Input: part model. Units: mm. Frame: model coordinates. A direction names the side the tool comes from. Coordinates: 2 decimals unless noted, no trailing zeros. Loops run counter-clockwise (first coordinate to the right, second up) from the corner with the lowest first, then second, coordinate; pieces in that order, holes last. Notation, with made-up numbers: (2, 78.5) -> (11, 78.5) arc R15 ccw to (11, 96.5) -> close; hole circle Ø1 at (18.25, 22.25). An arc over 180 degrees is marked (long way). Answer as a JSON object with one key per item and string values.
from build123d import *

# Parameters (mm, degrees)
ESQUISSE1_W                  = 41
ESQUISSE1_H                  = 46
ESQUISSE1_R                  = 2.25
ESQUISSE1_R_2                = 1
BOSS_EXTRU_1_DEPTH           = 30
ENL_V_START                  = 30
ESQUISSE2_W                  = 7
ESQUISSE2_H                  = 46
ENL_V_MAT_EXTRU_1_DEPTH      = 14
ENL_V_MAT_EXTRU_3_DEPTH      = 28.002906878
ENL_V_MAT_EXTRU_3_DEPTH_BACK = 44.002906878
ENL_V_MAT_EXTRU_3_START      = 16
ESQUISSE2_3_R                = 3
ESQUISSE3_W                  = 33.5
ESQUISSE3_H                  = 38
ENL_V_MAT_EXTRU_4_DEPTH      = 28
ESQUISSE4_W                  = 30
ESQUISSE4_H                  = 0.997507574
BOSS_EXTRU_2_DEPTH           = 1
CONG_1_R                     = 2
CONG_2_R                     = 2


# Some blends are built 0.0001 mm under size
with BuildPart() as part:
    # Esquisse1 → Boss.-Extru.1 (new body)
    with BuildSketch(Plane(origin=(0, 0, 0), x_dir=(1, 0, 0), z_dir=(0, 1, 0))):
        Rectangle(ESQUISSE1_W, ESQUISSE1_H)
        with Locations(Location((5.4, 0, 0), (0, 0, 270))):
            Circle(ESQUISSE1_R, mode=Mode.SUBTRACT)
        with Locations(Location((-1.85, 0, 0), (0, 0, 270))):
            Circle(ESQUISSE1_R_2, mode=Mode.SUBTRACT)
        with Locations(Location((12.65, 0, 0), (0, 0, 270))):
            Circle(ESQUISSE1_R_2, mode=Mode.SUBTRACT)
    extrude(amount=BOSS_EXTRU_1_DEPTH)

    # Esquisse2 → Enlèv. mat.-Extru.1 (cut)
    with BuildSketch(Plane(origin=(0, 0, 0), x_dir=(1, 0, 0), z_dir=(0, 1, 0)).offset(ENL_V_START)):
        with Locations((-17, 0)):
            Rectangle(ESQUISSE2_W, ESQUISSE2_H)
    extrude(amount=-ENL_V_MAT_EXTRU_1_DEPTH, mode=Mode.SUBTRACT)

    # Esquisse2<3> → Enlèv. mat.-Extru.3 (cut, two sides: drawn at the far end of the back side and taken through both)
    with BuildSketch(Plane(origin=(0, 0, 0), x_dir=(1, 0, 0), z_dir=(0, 1, 0)).offset(ENL_V_MAT_EXTRU_3_START - ENL_V_MAT_EXTRU_3_DEPTH_BACK)):
        with Locations(Location((-17, -8.75, 0), (0, 0, 90))):
            Circle(ESQUISSE2_3_R)
        with Locations(Location((-17, 8.75, 0), (0, 0, 90))):
            Circle(ESQUISSE2_3_R)
    extrude(amount=ENL_V_MAT_EXTRU_3_DEPTH + ENL_V_MAT_EXTRU_3_DEPTH_BACK, mode=Mode.SUBTRACT)

    # Esquisse3 → Enlèv. mat.-Extru.4 (cut)
    with BuildSketch(Plane(origin=(0, 0, 0), x_dir=(1, 0, 0), z_dir=(0, 1, 0))):
        with Locations((3.75, 0)):
            Rectangle(ESQUISSE3_W, ESQUISSE3_H)
    extrude(amount=ENL_V_MAT_EXTRU_4_DEPTH, mode=Mode.SUBTRACT)

    # Esquisse4 → Boss.-Extru.2 (add)
    with BuildSketch(Plane(origin=(0, 0, 0), x_dir=(1, 0, 0), z_dir=(0, 1, 0))):
        with Locations((5.5, -21)):
            Rectangle(ESQUISSE4_W, ESQUISSE4_H)
        with Locations((5.5, 21)):
            Rectangle(ESQUISSE4_W, ESQUISSE4_H)
    extrude(amount=-BOSS_EXTRU_2_DEPTH)

    # Congé1
    # the kernel refuses this fillet: 2 mm, written as the material it takes off along each edge
    with BuildSketch(Plane(origin=(-11.5, 28, -21), x_dir=(-1, 0, 0), z_dir=(0, 0, -1))) as cong_1_piece_1_section:
        Polygon((0, 0), (CONG_1_R, 0), (CONG_1_R, CONG_1_R), (0, CONG_1_R), align=None)
    cong_1_piece_1 = extrude(amount=CONG_1_R, mode=Mode.PRIVATE)
    cong_1_piece_1 = cong_1_piece_1 - Plane(origin=(-11.5, 28, -21), x_dir=(0.7071067811865475, -0.7071067811865475, 0), z_dir=(0, 0, -1)) * Sphere(CONG_1_R, mode=Mode.PRIVATE)
    add(cong_1_piece_1, mode=Mode.SUBTRACT)
    with BuildSketch(Plane(origin=(-18.5, 14, -21), x_dir=(0, 1, 0), z_dir=(-1, 0, 0))) as cong_1_piece_2_section:
        Polygon((0, 0), (CONG_1_R, 0), (CONG_1_R, CONG_1_R), (0, CONG_1_R), align=None)
    cong_1_piece_2 = extrude(amount=CONG_1_R, mode=Mode.PRIVATE)
    cong_1_piece_2 = cong_1_piece_2 - Plane(origin=(-18.5, 14, -21), x_dir=(0, -0.7071067811865475, 0.7071067811865475), z_dir=(-1, 0, 0)) * Sphere(CONG_1_R, mode=Mode.PRIVATE)
    add(cong_1_piece_2, mode=Mode.SUBTRACT)
    with BuildSketch(Plane(origin=(-11.5, 28, 21), x_dir=(-1, 0, 0), z_dir=(0, 0, 1))) as cong_1_piece_3_section:
        Polygon((0, 0), (CONG_1_R, 0), (CONG_1_R, -CONG_1_R), (0, -CONG_1_R), align=None)
    cong_1_piece_3 = extrude(amount=CONG_1_R, mode=Mode.PRIVATE)
    cong_1_piece_3 = cong_1_piece_3 - Plane(origin=(-11.5, 28, 21), x_dir=(0.7071067811865475, -0.7071067811865475, 0), z_dir=(0, 0, 1)) * Sphere(CONG_1_R, mode=Mode.PRIVATE)
    add(cong_1_piece_3, mode=Mode.SUBTRACT)
    with BuildSketch(Plane(origin=(-18.5, 14, 21), x_dir=(-1, 0, 0), z_dir=(0, 0, 1))) as cong_1_piece_4_section:
        Polygon((0, 0), (CONG_1_R, 0), (CONG_1_R, -CONG_1_R), (0, -CONG_1_R), align=None)
    cong_1_piece_4 = extrude(amount=CONG_1_R, mode=Mode.PRIVATE)
    cong_1_piece_4 = cong_1_piece_4 - Plane(origin=(-18.5, 14, 21), x_dir=(0.7071067811865475, -0.7071067811865475, 0), z_dir=(0, 0, 1)) * Sphere(CONG_1_R, mode=Mode.PRIVATE)
    add(cong_1_piece_4, mode=Mode.SUBTRACT)
    with BuildSketch(Plane(origin=(-11.5, 30, -23), x_dir=(0, 0, 1), z_dir=(1, 0, 0))) as cong_1_piece_5:
        with BuildLine():
            CenterArc((CONG_1_R, CONG_1_R), CONG_1_R, 180, 90)
            Line((0, CONG_1_R), (0, 0))
            Line((0, 0), (CONG_1_R, 0))
        make_face()
    extrude(amount=37, mode=Mode.SUBTRACT)
    with BuildSketch(Plane(origin=(-20.5, -5, -23), x_dir=(0, 0, 1), z_dir=(0, 1, 0)), Plane(origin=(-20.5, -5, 23), x_dir=(1, 0, 0), z_dir=(0, 1, 0))) as cong_1_piece_6:
        with BuildLine():
            CenterArc((CONG_1_R, CONG_1_R), CONG_1_R, 180, 90)
            Line((0, CONG_1_R), (0, 0))
            Line((0, 0), (CONG_1_R, 0))
        make_face()
    extrude(amount=19, mode=Mode.SUBTRACT)
    with BuildSketch(Plane(origin=(25.5, 30, 23), x_dir=(0, -1, 0), z_dir=(-1, 0, 0))) as cong_1_piece_7:
        with BuildLine():
            CenterArc((CONG_1_R, -CONG_1_R), CONG_1_R, 90, 90)
            Line((0, -CONG_1_R), (0, 0))
            Line((0, 0), (CONG_1_R, 0))
        make_face()
    extrude(amount=37, mode=Mode.SUBTRACT)
    with BuildSketch(Plane(origin=(-13.5, 16, 23), x_dir=(0, -1, 0), z_dir=(-1, 0, 0))) as cong_1_piece_8:
        with BuildLine():
            CenterArc((CONG_1_R, -CONG_1_R), CONG_1_R, 90, 90)
            Line((0, -CONG_1_R), (0, 0))
            Line((0, 0), (CONG_1_R, 0))
        make_face()
    extrude(amount=5, mode=Mode.SUBTRACT)
    with BuildSketch(Plane(origin=(-13.5, 28, 23), x_dir=(1, 0, 0), z_dir=(0, -1, 0)), Plane(origin=(-13.5, 28, -23), x_dir=(0, 0, 1), z_dir=(0, -1, 0))) as cong_1_piece_9:
        with BuildLine():
            CenterArc((CONG_1_R, -CONG_1_R), CONG_1_R, 90, 90)
            Line((0, -CONG_1_R), (0, 0))
            Line((0, 0), (CONG_1_R, 0))
        make_face()
    extrude(amount=12, mode=Mode.SUBTRACT)
    with BuildSketch(Plane(origin=(-20.5, 16, 21), x_dir=(0, -1, 0), z_dir=(0, 0, -1))) as cong_1_piece_10:
        with BuildLine():
            CenterArc((CONG_1_R, -CONG_1_R), CONG_1_R, 90, 90)
            Line((0, -CONG_1_R), (0, 0))
            Line((0, 0), (CONG_1_R, 0))
        make_face()
    extrude(amount=42, mode=Mode.SUBTRACT)
    with BuildSketch(Plane(origin=(-13.5, 30, -21), x_dir=(0, -1, 0), z_dir=(0, 0, 1))) as cong_1_piece_11:
        with BuildLine():
            CenterArc((CONG_1_R, CONG_1_R), CONG_1_R, 180, 90)
            Line((0, CONG_1_R), (0, 0))
            Line((0, 0), (CONG_1_R, 0))
        make_face()
    extrude(amount=42, mode=Mode.SUBTRACT)
    with BuildSketch(Plane(origin=(-18.5, 16, -23), x_dir=(0, 0, 1), z_dir=(1, 0, 0))) as cong_1_piece_12:
        with BuildLine():
            CenterArc((CONG_1_R, CONG_1_R), CONG_1_R, 180, 90)
            Line((0, CONG_1_R), (0, 0))
            Line((0, 0), (CONG_1_R, 0))
        make_face()
    extrude(amount=5, mode=Mode.SUBTRACT)
    with BuildSketch(Plane(origin=(-8.5, 16, 23), x_dir=(0, -1, 0), z_dir=(-1, 0, 0))) as cong_1_piece_13a_section:
        with BuildLine():
            CenterArc((CONG_1_R, -CONG_1_R), CONG_1_R, 90, 90)
            Line((0, -CONG_1_R), (0, 0))
            Line((0, 0), (CONG_1_R, 0))
        make_face()
    cong_1_piece_13a = extrude(amount=10, mode=Mode.PRIVATE)
    cong_1_piece_13a = split(cong_1_piece_13a, bisect_by=Plane(origin=(-13.5, 15.547209771, 22.547209771), z_dir=(1, 0, 0)), keep=Keep.TOP, mode=Mode.PRIVATE)
    with BuildSketch(Plane(origin=(-13.5, 28, 23), x_dir=(1, 0, 0), z_dir=(0, -1, 0))) as cong_1_piece_13b_section:
        with BuildLine():
            CenterArc((CONG_1_R, -CONG_1_R), CONG_1_R, 90, 90)
            Line((0, -CONG_1_R), (0, 0))
            Line((0, 0), (CONG_1_R, 0))
        make_face()
    cong_1_piece_13b = extrude(amount=17, mode=Mode.PRIVATE)
    cong_1_piece_13b = split(cong_1_piece_13b, bisect_by=Plane(origin=(-13.047209771, 16, 22.547209771), z_dir=(0, -1, 0)), keep=Keep.TOP, mode=Mode.PRIVATE)
    cong_1_piece_13 = cong_1_piece_13a & cong_1_piece_13b
    add(cong_1_piece_13, mode=Mode.SUBTRACT)
    with BuildSketch(Plane(origin=(-18.5, 16, -23), x_dir=(0, 0, 1), z_dir=(1, 0, 0))) as cong_1_piece_14a_section:
        with BuildLine():
            CenterArc((CONG_1_R, CONG_1_R), CONG_1_R, 180, 90)
            Line((0, CONG_1_R), (0, 0))
            Line((0, 0), (CONG_1_R, 0))
        make_face()
    cong_1_piece_14a = extrude(amount=10, mode=Mode.PRIVATE)
    cong_1_piece_14a = split(cong_1_piece_14a, bisect_by=Plane(origin=(-13.5, 15.547209771, -22.547209771), z_dir=(1, 0, 0)), keep=Keep.TOP, mode=Mode.PRIVATE)
    with BuildSketch(Plane(origin=(-13.5, 28, -23), x_dir=(0, 0, 1), z_dir=(0, -1, 0))) as cong_1_piece_14b_section:
        with BuildLine():
            CenterArc((CONG_1_R, -CONG_1_R), CONG_1_R, 90, 90)
            Line((0, -CONG_1_R), (0, 0))
            Line((0, 0), (CONG_1_R, 0))
        make_face()
    cong_1_piece_14b = extrude(amount=17, mode=Mode.PRIVATE)
    cong_1_piece_14b = split(cong_1_piece_14b, bisect_by=Plane(origin=(-13.047209771, 16, -22.547209771), z_dir=(0, -1, 0)), keep=Keep.TOP, mode=Mode.PRIVATE)
    cong_1_piece_14 = cong_1_piece_14a & cong_1_piece_14b
    add(cong_1_piece_14, mode=Mode.SUBTRACT)

    # Congé2
    cong_2_edges = [part.edges().sort_by_distance(p)[0] for p in [
        (20.5, 14, 23),
        (20.5, 29.414213562, 22.414213562),
        (20.5, 14, -23),
        (20.5, 29.414213562, -22.414213562),
        (20.5, 30, 0),
    ]]
    fillet(cong_2_edges, radius=CONG_2_R - 0.0001)  # a hair under: the kernel refuses the full size


solid = part.part
1. Section query B-B (x = 5.4). Return loops of the section in (y, z).
Reply:
{"outline": "(-1, -21.5) -> (0, -21.5) -> (0, -23) -> (28, -23) arc R2 ccw to (30, -21) -> (30, -2.25) -> (28, -2.25) -> (28, -19) -> (0, -19) -> (0, -20.5) -> (-1, -20.5) -> close; (-1, 20.5) -> (0, 20.5) -> (0, 19) -> (28, 19) -> (28, 2.25) -> (30, 2.25) -> (30, 21) arc R2 ccw to (28, 23) -> (0, 23) -> (0, 21.5) -> (-1, 21.5) -> close"}
2. Pin query (flat end, axial travel): P1, Ø12, axis at x = 1, z = 0.5, coming from the -Y side; P2, Ø0.8, axis at x = 0, y = -0.5, coming from the -Z side; P3, Ø1.5, axis at x = -15.5, z = 6.5, coming from the +Y side; P4, Ø4, axis at x = 5.4, z = 0, coming from the +Y side. Return the tip coordinate at first contact, or that it passes through.
Reply:
{"P1": "stops at y = 28", "P2": "stops at z = -21.5", "P3": "stops at y = 16", "P4": "passes through"}
3. Line query: line 1 along Z through (x, y) = (-17, 4); line 2 along Z through (x, y) = (13, 23.5); line 3 along X through (y, z) = (29.3, 0). Output: solid intervals per line, ascending.
Reply:
{"line 1": "z = -23 to -11.75, -5.75 to 5.75, 11.75 to 23", "line 2": "z = -23 to -19, 19 to 23", "line 3": "x = -13.02 to -2.85, -0.85 to 3.15, 7.65 to 11.65, 13.65 to 20.02"}
4. Section query A-A (z = 0). Count the separate pieces of the cut face and the enclosed holes in it, plus the area to 3 significant figures.
Reply:
{"separate pieces": "4", "enclosed holes": "0", "area": "174 mm2"}
5. Mould query, pull axis X, two halves, no side actions, for faces 4 (the face through (-14, 0, 2)), 5 (the face through (-2.826, 28.986, -0.217)), 6 (the face through (-12.9, 21.1, 22.43)). Classes: pulls with the +X half, pulls with the -X half, needs draft (parallel to the pull), parting line crosses it, or undercut.
Reply:
{"face 4": "needs draft", "face 5": "undercut", "face 6": "pulls with the -X half"}
6. Access query for faces 1 (the face through (0, 28, 0)), 2 (the face through (3.29, 29.4, -22.43)), 3 (the face through (-13.5, 22, 0)). Directions: +Z, -Z, +X, -X, +Y, -Y. A direction counts if a zero-diameter tool reaches every point of the face in a straight line with its end or side. Return the directions, or none.
Reply:
{"face 1": "+X, -Y", "face 2": "-Z, +X, -X, +Y", "face 3": "+Z, -Z, -X, +Y"}
7. Section query C-C (y = 25.5). Return loops of the section in (x, z).
Reply:
{"outline": "(-13.5, -21) arc R2 ccw to (-11.5, -23) -> (18.5, -23) arc R2 ccw to (20.5, -21) -> (20.5, -19) -> (-13, -19) -> (-13, 19) -> (20.5, 19) -> (20.5, 21) arc R2 ccw to (18.5, 23) -> (-11.5, 23) arc R2 ccw to (-13.5, 21) -> close"}
